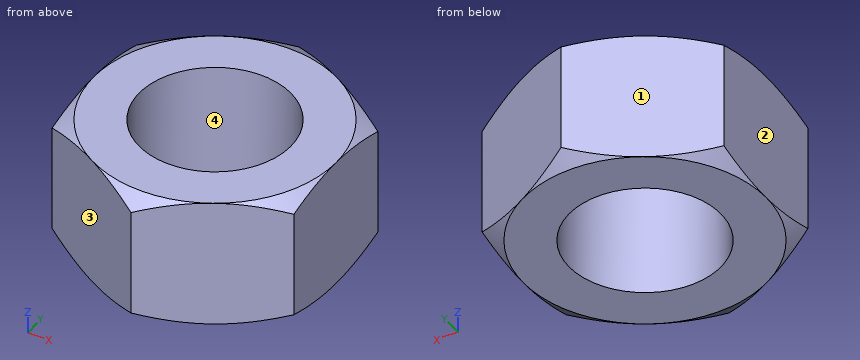
from build123d import *

# Parameters (mm, degrees)
SKETCH1_R               = 3.96875
EXTRUDE1_DEPTH          = 3.3734375
SKETCH7_OUTSIDE_W       = 106.796
SKETCH7_OUTSIDE_H       = 108.76
SKETCH7_OUTSIDE_R       = 6.35
EXTRUDE2_DEPTH          = 25.4
EXTRUDE2_DRAFT          = -60
MIRROR1_COPY_1_SKETCH_W = 106.796
MIRROR1_COPY_1_SKETCH_H = 108.76
MIRROR1_COPY_1_SKETCH_R = 6.35
MIRROR1_COPY_1_DEPTH    = 25.4
MIRROR1_COPY_1_DRAFT    = -60


with BuildPart() as part:
    # Sketch1 → Extrude1 (new, symmetric)
    with BuildSketch(Plane.XY):
        Polygon((-6.35, 3.666174209), (-6.35, -3.666174209), (0, -7.332348419), (6.35, -3.666174209), (6.35, 3.666174209), (0, 7.332348419), align=None)
        Circle(SKETCH1_R, mode=Mode.SUBTRACT)
    extrude(amount=EXTRUDE1_DEPTH, both=True)


with BuildPart() as extrude2_tool:
    # Sketch7 outside → Extrude2 (with draft: the straight prism first)
    with BuildSketch(Plane.XY.offset(3.3734375)):
        Rectangle(SKETCH7_OUTSIDE_W, SKETCH7_OUTSIDE_H)
        Circle(SKETCH7_OUTSIDE_R, mode=Mode.SUBTRACT)
    extrude(amount=-EXTRUDE2_DEPTH)
    # Extrude2: the draft: its side faces are tilted about the plane it starts from
    extrude2_sides = [extrude2_tool.faces().sort_by_distance(p)[0] for p in [
        (0, -54.38, -9.3265625),
        (53.398, 0, -9.3265625),
        (0, 54.38, -9.3265625),
        (-53.398, 0, -9.3265625),
        (-6.35, 0, -9.3265625),
    ]]
    draft(extrude2_sides, Plane.XY.offset(3.3734375), EXTRUDE2_DRAFT)


with BuildPart() as part_1:
    add(part.part)

    # Extrude2: cut by extrude2_tool
    add(extrude2_tool.part, mode=Mode.SUBTRACT)


with BuildPart() as mirror1_copy_1_tool:
    # Mirror1 copy 1 sketch → Mirror1 copy 1 (with draft: the straight prism first)
    with BuildSketch(Plane(origin=(0, 0, -3.3734375), x_dir=(1, 0, 0), z_dir=(0, 0, -1))):
        Rectangle(MIRROR1_COPY_1_SKETCH_W, MIRROR1_COPY_1_SKETCH_H)
        Circle(MIRROR1_COPY_1_SKETCH_R, mode=Mode.SUBTRACT)
    extrude(amount=-MIRROR1_COPY_1_DEPTH)
    # Mirror1 copy 1: the draft: its side faces are tilted about the plane it starts from
    mirror1_copy_1_sides = [mirror1_copy_1_tool.faces().sort_by_distance(p)[0] for p in [
        (0, -54.38, 9.3265625),
        (53.398, 0, 9.3265625),
        (0, 54.38, 9.3265625),
        (-53.398, 0, 9.3265625),
        (-6.35, 0, 9.3265625),
    ]]
    draft(mirror1_copy_1_sides, Plane(origin=(0, 0, -3.3734375), x_dir=(1, 0, 0), z_dir=(0, 0, -1)), MIRROR1_COPY_1_DRAFT)


with BuildPart() as part_2:
    add(part_1.part)

    # Mirror1 copy 1: cut by mirror1_copy_1_tool
    add(mirror1_copy_1_tool.part, mode=Mode.SUBTRACT)


solid = part_2.part
Could you check a few things on this model? Use its own coordinates, in mm. Face numbers are marked on the shaded views. Give positions to 0.01 mm unless a question says otherwise; leave off trailing zeros. Order: outer loops, then holes, each group sorted by start corner. A loop starts at its lowest first (then second) coordinate and runs counter-clockwise, first axis right, second up.
1. I need wall thicknesses on L1, parallel to Y at x = -0.5, z = 2.75; L2, parallel to X at y = -3.25, z = -1.75; L3, parallel to Y at x = 2.75, z = -1.5. Which ranges of each line are inside material? Lowest first, please.
Answers below:
L1: y = -7.04 to -3.94, 3.94 to 7.04
L2: x = -6.35 to -2.28, 2.28 to 6.35
L3: y = -5.74 to -2.86, 2.86 to 5.74
2. Thinking about a two-plate mould opening in Y: for the marked faces 1, 2, 3 and 4, which applies, +Y half, -Y half, draft (parallel to the pull), parting line (faces both ways), or undercut?
Answers below:
face 1: +Y half
face 2: draft
face 3: -Y half
face 4: undercut
3. Suppose I cut it at A-A (z = 0.75). Write out the boundary of the cut face in (x, y).
Answers below:
outline: (-6.35, -3.67) - (0, -7.33) - (6.35, -3.67) - (6.35, 3.67) - (0, 7.33) - (-6.35, 3.67) - close; hole circle Ø7.94 at (0, 0)
4. For pin 1 (4 mm diameter, centred on y = -4, z = 0.5, fed in from +X), with a flat end and sliding along its axis, tell me the tip position at first contact or that it passes through.
Answers below:
pin 1: stops at x = 6.35
